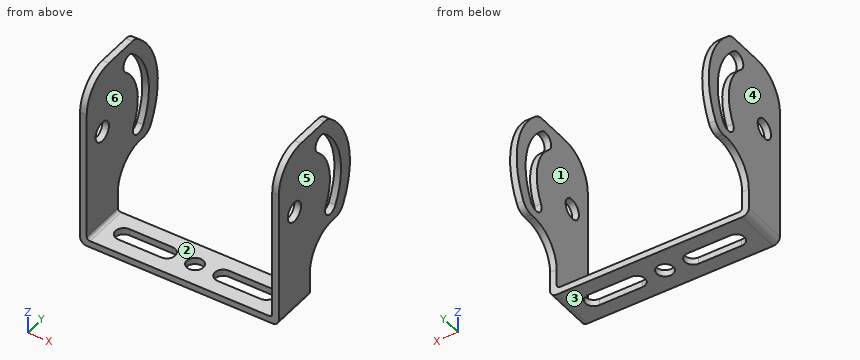
from build123d import *

# Parameters (mm, degrees)
F0_R     = 1.5
F1_DEPTH = 15
F3_DEPTH = 25
F4_R     = 1
F5_R     = 1.25
F6_DEPTH = 25


with BuildPart() as f1:
    # F0 (on Right) → F1 (new body, symmetric)
    with BuildSketch(Plane.YZ):
        with BuildLine():
            Line((-3.5, 21), (-3.5, 0))
            Line((-3.5, 0), (3.5, 0))
            Line((3.5, 0), (3.5, 4))
            ThreePointArc((3.5, 4), (4.964466, 7.535534), (8.5, 9))
            Line((8.5, 9), (9.233093, 9))
            ThreePointArc((9.233093, 9), (10.256625, 9.281751), (10.991777, 10.047619))
            ThreePointArc((10.991777, 10.047619), (12.286782, 18.298911), (8.096113, 25.52381))
            ThreePointArc((8.096113, 25.52381), (7.490801, 25.877181), (6.800735, 26))
            Line((6.800735, 26), (1.5, 26))
            ThreePointArc((1.5, 26), (-2.035534, 24.535534), (-3.5, 21))
        make_face()
        with Locations((0, 16)):
            Circle(F0_R, mode=Mode.SUBTRACT)
        with BuildLine():
            ThreePointArc((6.800735, 24), (10.320897, 17.931085), (9.233093, 11))
            ThreePointArc((9.233093, 11), (7.538677, 10.49606), (7.034737, 12.190476))
            ThreePointArc((7.034737, 12.190476), (7.86354, 17.471303), (5.181513, 22.095238))
            ThreePointArc((5.181513, 22.095238), (5.038743, 23.85723), (6.800735, 24))
        make_face(mode=Mode.SUBTRACT)
    extrude(amount=F1_DEPTH, both=True)

    # F2 (on face) → F3 (cut)
    with BuildSketch(Plane.XZ.offset(3.5)):
        with BuildLine():
            Line((14, 26), (-14, 26))
            Line((-14, 26), (-14, 1.5))
            ThreePointArc((-14, 1.5), (-13.853553, 1.146447), (-13.5, 1))
            Line((-13.5, 1), (13.5, 1))
            ThreePointArc((13.5, 1), (13.853553, 1.146447), (14, 1.5))
            Line((14, 1.5), (14, 26))
        make_face()
    extrude(amount=-F3_DEPTH, mode=Mode.SUBTRACT)

    # F4
    f4_edges = [f1.edges().sort_by_distance(p)[0] for p in [
        (-15, 0, 0),
        (15, 0, 0),
    ]]
    fillet(f4_edges, radius=F4_R)

    # F5 (on face) → F6 (cut)
    with BuildSketch(Plane(origin=(0, 0, 0), x_dir=(1, 0, 0), z_dir=(0, 0, -1))):
        Circle(F5_R)
        with BuildLine():
            ThreePointArc((-10.75, 1.25), (-12, 0), (-10.75, -1.25))
            Line((-10.75, -1.25), (-4.25, -1.25))
            ThreePointArc((-4.25, -1.25), (-3, 0), (-4.25, 1.25))
            Line((-4.25, 1.25), (-10.75, 1.25))
        make_face()
        with BuildLine():
            ThreePointArc((10.75, -1.25), (12, 0), (10.75, 1.25))
            Line((10.75, 1.25), (4.25, 1.25))
            ThreePointArc((4.25, 1.25), (3, 0), (4.25, -1.25))
            Line((4.25, -1.25), (10.75, -1.25))
        make_face()
    extrude(amount=-F6_DEPTH, mode=Mode.SUBTRACT)


solid = f1.part
For this review, take the finished solid that the model builds, in its own axes (mm). Face numbers are marked on the shaded views. A direction names the side the tool comes from. Round coordinates to 2 decimals unless told otherwise and drop trailing zeros. Order: outer loops, then holes, each group sorted by start corner. A loop starts at its lowest first (then second) coordinate and runs counter-clockwise, first axis right, second up. Notation, with made-up numbers: (-4.5, 43) -> (28.5, 43) arc R19 cw to (28.5, 76) -> close; hole circle Ø9 at (-31, 73.25). An arc over 180 degrees is marked (long way). Write item = value, one per line. Start each with the question number.
1) Take a section at C-C on y = 7.5. State the section outline as (x, z) points, plus the area to 3 significant figures.
2) Tool access review of the marked faces 5 and 6: name each direction out of +Z, -Z, +X, -X, +Y, -Y from which nothing blocks a thin tool from reaching the whole face with its end or side.
3) The part is to be moulded in two halves that separate along X. For the marked faces 1, 2, 3 and 4, say which applies: +X half, -X half, draft (parallel to the pull), parting line (faces both ways), or undercut.
4) Take a section at A-A on x = 0. State the section outline as (y, z) points.
5) To check wall thickness, follow line 1 (Y direction, x = 14.25, z = 16); line 2 (Y direction, x = 0, z = 0.5); line 3 (X direction, y = 1.25, z = 5.25). State the ranges of each line that lie inside material, in increasing order. Write a range as from..to.
6) Take a section at D-D on z = 19.25. State the section outline as (x, y) points, plus the area to 3 significant figures.
7) Take a section at B-B on y = 11.75. State the section outline as (x, z) points, plus the area to 3 significant figures.
8) Insertion check: pin 1 (3.5 mm diameter, centred on y = 0, z = 16, fed in from -X); pin 2 (2 mm diameter, centred on x = 4.5, y = 0.5, fed in from +Z); pin 3 (0.8 mm diameter, centred on x = -14.5, y = 8.5, fed in from -Z); pin 4 (2 mm diameter, centred on x = 1, z = 1.5, fed in from +Y). Each pin has a flat end and moves straight along its axis. Give the tip position at first contact, or say it passes through.
Verdict:
q1.outline = (-15, 8.9) -> (-14, 8.9) -> (-14, 10.52) -> (-15, 10.52) -> close; (-15, 13.22) -> (-14, 13.22) -> (-14, 18.78) -> (-15, 18.78) -> close; (-15, 23.35) -> (-14, 23.35) -> (-14, 25.87) -> (-15, 25.87) -> close; (14, 8.9) -> (15, 8.9) -> (15, 10.52) -> (14, 10.52) -> close; (14, 13.22) -> (15, 13.22) -> (15, 18.78) -> (14, 18.78) -> close; (14, 23.35) -> (15, 23.35) -> (15, 25.87) -> (14, 25.87) -> close
q1.area = 19.4 mm2
q2.face_5 = +Z, -Z, +X, +Y, -Y
q2.face_6 = +Z, +Y, -Y
q3.face_1 = undercut
q3.face_2 = undercut
q3.face_3 = draft
q3.face_4 = -X half
q4.outline = (-3.5, 0) -> (-1.25, 0) -> (-1.25, 1) -> (-3.5, 1) -> close; (1.25, 0) -> (3.5, 0) -> (3.5, 1) -> (1.25, 1) -> close
q5.line_1 = -3.5..-1.5, 1.5..8, 10.5..12.5
q5.line_2 = -3.5..-1.25, 1.25..3.5
q5.line_3 = -15..-14, 14..15
q6.outline = (-15, -3.5) -> (-14, -3.5) -> (-14, 7.31) -> (-15, 7.31) -> close; (-15, 9.98) -> (-14, 9.98) -> (-14, 12.07) -> (-15, 12.07) -> close; (14, -3.5) -> (15, -3.5) -> (15, 7.31) -> (14, 7.31) -> close; (14, 9.98) -> (15, 9.98) -> (15, 12.07) -> (14, 12.07) -> close
q6.area = 25.8 mm2
q7.outline = (-15, 11.74) -> (-14, 11.74) -> (-14, 20.26) -> (-15, 20.26) -> close; (14, 11.74) -> (15, 11.74) -> (15, 20.26) -> (14, 20.26) -> close
q7.area = 17.1 mm2
q8.pin_1 = -15
q8.pin_2 = 1
q8.pin_3 = 8.98
q8.pin_4 = 3.5
